Work out the finished part from the listing and answer in its coordinate system (mm). Face numbers are marked on the shaded views. A direction names the side the tool comes from. Give positions to 0.01 mm unless a question says otherwise; leave off trailing zeros. Return JSON: item names as keys, results as strings. Group by question number.
from build123d import *

# Parameters (mm, degrees)
F_6_CLEARANCE_HOLE1_D     = 3.7973
F_6_CLEARANCE_HOLE1_DEPTH = 25.4
F_6_CLEARANCE_HOLE1_TIP   = 1.140824014


with BuildPart() as part:
    # Sketch1 → Revolve1 (revolve)
    with BuildSketch(Plane(origin=(0, 0, 0), x_dir=(1, 0, 0), z_dir=(0, 1, 0))):
        Polygon((0, 0), (88.9, 0), (88.9, -6.35), (77.6478, -6.35), (77.6478, -3.7084), (73.025, -3.7084), (73.025, -6.35), (69.723, -6.35), (69.723, -11.176), (66.6242, -11.176), (66.6242, -15.113), (69.723, -15.113), (69.723, -18.288), (66.6242, -18.288), (66.6242, -22.225), (69.723, -22.225), (69.723, -25.4), (63.4492, -25.4), (63.4492, -3.811809937), (0, -3.811809937), align=None)
    revolve(axis=Axis((0, 0, 0), (0, 0, 1)))

    # #6 Clearance Hole1
    with Locations(Plane.XY.offset(6.35)):
        with Locations((0, -83.2739), (79.198185232, -25.733050288), (48.947170321, 67.370000288), (-79.198185232, -25.733050288), (-48.947170321, 67.370000288)):
            Hole(F_6_CLEARANCE_HOLE1_D / 2, depth=F_6_CLEARANCE_HOLE1_DEPTH)
            with Locations((0, 0, -(F_6_CLEARANCE_HOLE1_DEPTH + F_6_CLEARANCE_HOLE1_TIP / 2))):  # 118° drill point
                Cone(0, F_6_CLEARANCE_HOLE1_D / 2, F_6_CLEARANCE_HOLE1_TIP, mode=Mode.SUBTRACT)


solid = part.part
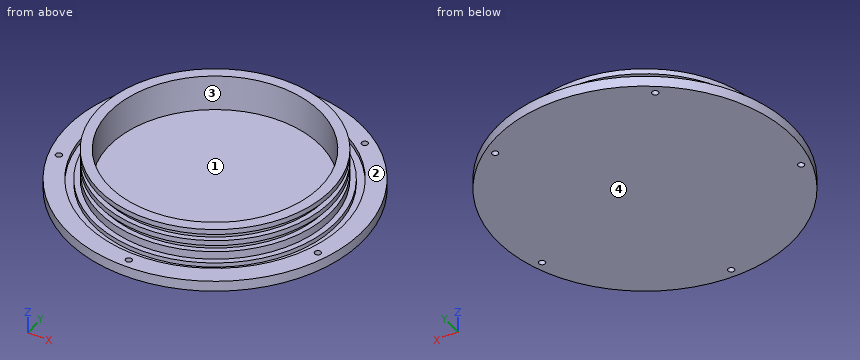
1. Each of these flat-tipped pins is pushed along its axis until it touches: pin 1 (10 mm diameter, centred on x = -41.5, y = -64.5, fed in from -Z); pin 2 (4 mm diameter, centred on y = 36, z = 19, fed in from +X); pin 3 (3 mm diameter, centred on x = 0, y = -83.27, fed in from +Z); pin 4 (5 mm diameter, centred on x = 71, y = -26, fed in from +Z). Where does it stop, or does it pass through?
2. Consider probe 1 along Z at (x, y) = (55, 40) (3 decimals); probe 2 along Y at (x, z) = (0, 5.65) (3 decimals); probe 3 along Y at (x, z) = (0, 2.75). Determine where each line is inside the solid, lowest interval first. Write a range as from..to.
3. A tool of negligible diameter and unlimited length cuts with its end or side. For the marked faces 3 and 4, from which of +Z, -Z, +X, -X, +Y, -Y can it reach the whole face along a straight path? Write none if from no direction.
4. Determine the mould class of the marked faces 1 and 2 for opening direction X: released by +X, released by -X, zero draft, split by the parting line, or undercut.
Answers:
{
 "1": {"pin 1": "stops at z = 0", "pin 2": "stops at x = 60.8", "pin 3": "passes through", "pin 4": "stops at z = 6.35"},
 "2": {"probe 1": "z = 0..11.176, 15.113..18.288, 22.225..25.4", "probe 2": "y = -88.9..-85.173, -81.375..-77.648, -73.025..-63.449, 63.449..73.025, 77.648..88.9", "probe 3": "y = -88.9..-85.17, -81.38..88.9"},
 "3": {"face 3": "+Z", "face 4": "-Z, +X, -X, +Y, -Y"},
 "4": {"face 1": "undercut", "face 2": "zero draft"}
}
